Autodesk Fusion 360 part; units mm, degrees
sketch "Sketch1" plane through (0, 0, 0) normal (1, 0, 0) x (0, 1, 0)
  line L0 (0, 0) -> (100, 0)
  line L1 (100, 0) -> (100, 15)
  line L2 (100, 15) -> (0, 15)
  line L3 (0, 15) -> (0, 0)
  dimension "d1" = 100
  dimension "d2" = 15
extrude "Extrude1" add sketch "Sketch1" along normal blind 6
sketch "Sketch2" plane through (6, 0, 0) normal (1, 0, 0) x (0, 1, 0)
  line L0 (0, 15) -> (0, 0)
  line L1 (0, 0) -> (100, 0)
  line L2 (100, 0) -> (100, 15)
  line L3 (100, 15) -> (0, 15)
  circle A0 centre (6, 7.5) radius 4
  circle A1 centre (94, 7.5) radius 4
  line L4 (6, 11.5) -> (94, 11.5)
  line L5 (94, 3.5) -> (6, 3.5)
  circle A2 centre (6, 7.5) radius 6.5013
  dimension "d5" = 8
  dimension "d6" = 6
  dimension "d7" = 8
  dimension "d8" = 6
extrude "Extrude2" cut sketch "Sketch2" against normal blind 20 contours A1 L4 L5 A2 | A0 | A1
sketch "Sketch3" plane through (0, 0, 0) normal (-1, 0, 0) x (0, -1, 0)
  line L0 (-11.1251, 3.5) -> (-94, 3.5)
  arc A0 (-94, 11.5) -> (-94, 3.5) centre (-94, 7.5) ccw
  line L1 (-94, 11.5) -> (-11.1251, 11.5)
  line L2 (0, 0) -> (0, 15)
  line L3 (0, 15) -> (-100, 15)
  line L4 (-100, 15) -> (-100, 0)
  line L5 (-100, 0) -> (0, 0)
  circle A1 centre (-6, 7.5) radius 4
  arc A2 (-11.1251, 11.5) -> (-11.1251, 3.5) centre (-6, 7.5) ccw
sketch "Sketch4" plane through (0, 50, 7.5) normal (-1, 0, 0) x (0, -1, 0)
sketch "Sketch5" plane through (0, 0, 0) normal (0, 0, -1) x (1, 0, 0)
  line L0 (0, 0) -> (0, -100)
  line L1 (0, -100) -> (6, -100)
  line L2 (6, -100) -> (6, 0)
  line L3 (6, 0) -> (0, 0)
  line L4 (0, -100) -> (-5, -100)
  line L5 (-5, -100) -> (-5, -95)
  line L6 (-5, -95) -> (0, -95)
  line L7 (0, -95) -> (0, -100)
  line L8 (0, 0) -> (-5, 0)
  line L9 (-5, 0) -> (-5, -5)
  line L10 (-5, -5) -> (0, -5)
  line L11 (0, -5) -> (0, 0)
  dimension "d11" = 5
  dimension "d12" = 5
  dimension "d13" = 5
  dimension "d14" = 5
extrude "Extrude3" add sketch "Sketch5" against normal blind 3 contours L0 L8 L9 L10 L11 | L0 L4 L5 L6 L7
sketch "Sketch6" plane through (0, 0, 3) normal (0, 0, 1) x (-1, 0, 0)
  line L0 (5, -95) -> (0, -95)
  line L1 (0, -95) -> (0, -100)
  line L2 (0, -100) -> (5, -100)
  line L3 (5, -100) -> (5, -95)
  circle A0 centre (2.5, -97.5) radius 2
  dimension "d17" = 4
extrude "Extrude4" cut sketch "Sketch6" against normal blind 6 contours A0
sketch "Sketch7" plane through (0, 0, 0) normal (-1, 0, 0) x (0, -1, 0)
sketch "Sketch8" plane through (0, 0, 3) normal (0, 0, 1) x (-1, 0, 0)
  line L0 (0, 0) -> (0, -5)
  line L1 (0, -5) -> (5, -5)
  line L2 (5, -5) -> (5, 0)
  line L3 (5, 0) -> (0, 0)
  circle A0 centre (2.5, -2.5) radius 2
  dimension "d20" = 4
extrude "Extrude5" cut sketch "Sketch8" against normal blind 9 contours A0
sketch "Sketch9" plane through (0, 50.3094, 7.5) normal (-1, 0, 0) x (0, -1, 0)
extrude "Extrude6" add 1 faces at (4, 65, 0) along direction (0, 0, -1) blind 20
sketch "Sketch10" plane through (0, 0, 0) normal (-1, 0, 0) x (0, -1, 0)
  line L0 (-5, 3) -> (0, 3)
  line L1 (0, 3) -> (0, 15)
  line L2 (0, 15) -> (-100, 15)
  line L3 (-100, 15) -> (-100, 3)
  line L4 (-100, 3) -> (-95, 3)
  line L5 (-95, 3) -> (-95, -20)
  line L6 (-95, -20) -> (-5, -20)
  line L7 (-5, -20) -> (-5, 3)
  circle A0 centre (-6, 7.5) radius 4
  line L8 (-94, 11.5) -> (-11.1251, 11.5)
  arc A1 (-11.1251, 11.5) -> (-11.1251, 3.5) centre (-6, 7.5) ccw
  line L9 (-11.1251, 3.5) -> (-94, 3.5)
  arc A2 (-94, 11.5) -> (-94, 3.5) centre (-94, 7.5) ccw
  line L10 (-95, -20) -> (-50, 0)
  line L11 (-50, 0) -> (-5, -20)
extrude "Extrude7" cut sketch "Sketch10" against normal blind 25 contours L6 L10 L11
fillet "Fillet1" radius 25 1 edges at (3, 50, 0)
sketch "Sketch11" plane through (6, 0, 0) normal (1, 0, 0) x (0, 1, 0)
  line L0 (5, -20) -> (39.8465, -4.5126)
  arc A0 (60.1535, -4.5126) -> (39.8465, -4.5126) centre (50, -27.3579) ccw
  line L1 (60.1535, -4.5126) -> (95, -20)
  line L2 (95, -20) -> (100, -20)
  line L3 (100, -20) -> (100, 15)
  line L4 (100, 15) -> (0, 15)
  line L5 (0, 15) -> (0, -20)
  line L6 (0, -20) -> (5, -20)
  line L7 (11.1251, 11.5) -> (94, 11.5)
  arc A1 (94, 3.5) -> (94, 11.5) centre (94, 7.5) ccw
  line L8 (94, 3.5) -> (11.1251, 3.5)
  arc A2 (11.1251, 3.5) -> (11.1251, 11.5) centre (6, 7.5) ccw
  circle A3 centre (6, 7.5) radius 4
  circle A4 centre (6, 7.5) radius 2
  circle A5 centre (94, 7.5) radius 2
  line L9 (94, 9.5) -> (12.186, 9.5)
  line L10 (94, 5.5) -> (12.186, 5.5)
  dimension "d29" = 4
  dimension "d30" = 4
extrude "Extrude8" add sketch "Sketch11" against normal blind 6 contours L7 A1 L8 A2 A5 L9 L10 | A3
Geometry: final body of the model. Coordinates: model frame, mm. A direction names the side the tool comes from. Coordinates: 2 decimals unless noted, no trailing zeros. Order: outer loops, then holes, each group sorted by start corner. A loop starts at its lowest first (then second) coordinate and runs counter-clockwise, first axis right, second up. Notation, with made-up numbers: (-22.75, 30.25) - (-18.75, 30.25) arc R24 ccw to (-18.75, 43.25) - close; hole circle Ø3 at (-20, 65.25). An arc over 180 degrees is marked (long way). Write each question's results on one line, items separated by ' | '.
1) Pin query (flat end, axial travel): pin 1 (1.5 mm diameter, centred on x = -2, y = 47, fed in from -Z); pin 2 (3 mm diameter, centred on x = 3.5, y = 35, fed in from -Z); pin 3 (1.5 mm diameter, centred on x = 5, y = 75.5, fed in from -Z); pin 4 (1 mm diameter, centred on x = 4.5, y = 20, fed in from -Z). Return the tip coordinate at first contact, or that it passes through.
Results list:
pin 1: through | pin 2: z = -7.33 | pin 3: z = -11.67 | pin 4: z = -13.56
2) Section D-D, the plane y = 27. Return loops of the section in (x, z), plus the area to 3 significant figures.
Results list:
outline: (0, -10.22) - (6, -10.22) - (6, 5.5) - (0, 5.5) - close; (0, 9.5) - (6, 9.5) - (6, 15) - (0, 15) - close | area: 127 mm^2
3) Line query: line 1 (Y direction, x = -2.75, z = -10); line 2 (X direction, y = 2.5, z = -4.75); line 3 (Y direction, x = 2.75, z = 7). Output: solid intervals per line, ascending. Write a range as from..to.
Results list:
line 1: 0..0.52, 4.48..5, 95..95.52, 99.48..100 | line 2: -5..-4.5, -0.5..6 | line 3: 0..4.06, 7.94..12.48, 95.94..100
4) Section B-B, the plane x = -2.5. Return loops of the section in (y, z).
Results list:
outline: (0, -20) - (0.5, -20) - (0.5, 3) - (0, 3) - close; (4.5, -20) - (5, -20) - (5, 3) - (4.5, 3) - close; (95, -20) - (95.5, -20) - (95.5, 3) - (95, 3) - close; (99.5, -20) - (100, -20) - (100, 3) - (99.5, 3) - close
5) Section A-A, the plane y = 2.5. Return loops of the section in (x, z).
Results list:
outline: (-5, -20) - (-4.5, -20) - (-4.5, 3) - (-5, 3) - close; (-0.5, -20) - (6, -20) - (6, 15) - (0, 15) - (0, 3) - (-0.5, 3) - close
6) Pull-direction query (X, two-part tool) for faces 6 (the cylindrical face through (-2.066, 4.452, -8.339)), 7 (the cylindrical face through (-2.24, 95.517, -8.339)), 8 (the flat face through (-5, 98, -8)), 9 (the flat face through (0, 0, -6)); classes: pulls with the +X half, pulls with the -X half, needs draft (parallel to the pull), parting line crosses it, or undercut.
Results list:
face 6: undercut | face 7: undercut | face 8: pulls with the -X half | face 9: needs draft
7) Section C-C, the plane x = 2.75. Return loops of the section in (y, z), plus the area to 3 significant figures.
Results list:
outline: (0, -20) - (5, -20) - (39.85, -4.51) arc R25 cw to (60.15, -4.51) - (95, -20) - (100, -20) - (100, 15) - (0, 15) - close; hole circle Ø4 at (6, 7.5); hole (12.19, 5.5) - (94, 5.5) arc R2 ccw to (94, 9.5) - (12.19, 9.5) arc R6.5 cw to start | area: 2,270 mm^2
8) Set-up query: faces 1 (the flat face through (3, 23, -12)), 2 (the flat face through (-4.8, 2.5, 3)), 3 (the flat face through (-3, 5, -8)), 4 (the flat face through (6, 49, -2)), 5 (the flat face through (3, 54, 9.5)). Return all of +Z, -Z, +X, -X, +Y, -Y with unobstructed straight access to the full face (end or side cutting, diameter ignored); none if empty.
Results list:
face 1: -Z, +X, -X | face 2: +Z, -X, +Y, -Y | face 3: +Z, -Z, -X | face 4: +Z, -Z, +X, +Y, -Y | face 5: +X, -X
